Geometry check sheet. Reference: the model listing, model coordinates, mm. A direction names the side the tool comes from. Round coordinates to 2 decimals unless told otherwise and drop trailing zeros. Write each loop counter-clockwise with the first axis right and the second up, starting at its lowest first coordinate (ties: lowest second). Pieces come first, ordered by that corner, then holes. Notation, with made-up numbers: (81, -8.5) - (104, -8.5) arc R11 ccw to (104, 3.5) - close; hole circle Ø6 at (59, 6.5). An arc over 180 degrees is marked (long way). Return JSON: item names as keys, results as strings.
```python
from build123d import *

# Parameters (mm, degrees)
SKETCH1_R           = 23
SKETCH1_R_2         = 1.6
BOSS_EXTRUDE1_DEPTH = 10
SKETCH2_R           = 27.6
CUT_EXTRUDE1_DEPTH  = 7


with BuildPart() as part:
    # Sketch1 → Boss-Extrude1 (new body)
    with BuildSketch(Plane.XY):
        with BuildLine():
            ThreePointArc((-28.945945946, 19.675675676), (-35, 0), (-28.945945946, -19.675675676))
            ThreePointArc((-28.945945946, -19.675675676), (-28.600540614, -20.846499055), (-29, -22))
            ThreePointArc((-29, -22), (-28.535533906, -28.535533906), (-22, -29))
            ThreePointArc((-22, -29), (-20.846499055, -28.600540614), (-19.675675676, -28.945945946))
            ThreePointArc((-19.675675676, -28.945945946), (0, -35), (19.675675676, -28.945945946))
            ThreePointArc((19.675675676, -28.945945946), (20.846499055, -28.600540614), (22, -29))
            ThreePointArc((22, -29), (28.535533906, -28.535533906), (29, -22))
            ThreePointArc((29, -22), (28.600540614, -20.846499055), (28.945945946, -19.675675676))
            ThreePointArc((28.945945946, -19.675675676), (35, 0), (28.945945946, 19.675675676))
            ThreePointArc((28.945945946, 19.675675676), (28.600540614, 20.846499055), (29, 22))
            ThreePointArc((29, 22), (28.535533906, 28.535533906), (22, 29))
            ThreePointArc((22, 29), (20.846499055, 28.600540614), (19.675675676, 28.945945946))
            ThreePointArc((19.675675676, 28.945945946), (0, 35), (-19.675675676, 28.945945946))
            ThreePointArc((-19.675675676, 28.945945946), (-20.846499055, 28.600540614), (-22, 29))
            ThreePointArc((-22, 29), (-28.535533906, 28.535533906), (-29, 22))
            ThreePointArc((-29, 22), (-28.600540614, 20.846499055), (-28.945945946, 19.675675676))
        make_face()
        Circle(SKETCH1_R, mode=Mode.SUBTRACT)
        with Locations((-25, 25)):
            Circle(SKETCH1_R_2, mode=Mode.SUBTRACT)
        with Locations((25, 25)):
            Circle(SKETCH1_R_2, mode=Mode.SUBTRACT)
        with Locations((-25, -25)):
            Circle(SKETCH1_R_2, mode=Mode.SUBTRACT)
        with Locations((25, -25)):
            Circle(SKETCH1_R_2, mode=Mode.SUBTRACT)
    extrude(amount=BOSS_EXTRUDE1_DEPTH)

    # Sketch2 → Cut-Extrude1 (cut)
    with BuildSketch(Plane.XY.offset(10)):
        Circle(SKETCH2_R)
    extrude(amount=-CUT_EXTRUDE1_DEPTH, mode=Mode.SUBTRACT)


solid = part.part
```
(1) Release check for a two-part mould opening along Y. For faces 1 (the face through (0, 35, 5)), 2 (the face through (-28, 29, 5)), 3 (the face through (-29, -28, 5)), 4 (the face through (-20.86, -28.6, 4.93)) record: pulls with the +Y half, pulls with the -Y half, needs draft (parallel to the pull), parting line crosses it, or undercut.
Response values:
{"face 1": "pulls with the +Y half", "face 2": "undercut", "face 3": "undercut", "face 4": "pulls with the -Y half"}
(2) Section check C-C, the plane y = 25. Enter the section's corners in (x, z).
Response values:
{"outline": "(-30, 0) - (-26.6, 0) - (-26.6, 10) - (-30, 10) - close; (-23.4, 0) - (23.4, 0) - (23.4, 10) - (11.69, 10) - (11.69, 3) - (-11.69, 3) - (-11.69, 10) - (-23.4, 10) - close; (26.6, 0) - (30, 0) - (30, 10) - (26.6, 10) - close"}
(3) Gauge pin test, flat ends, axial feed: pin 1 (3 mm diameter, centred on x = 8.5, z = 3, fed in from -Y); pin 2 (2 mm diameter, centred on y = 13, z = 7.5, fed in from -X); pin 3 (1 mm diameter, centred on x = 1, y = -25.5, fed in from +Z). Record the tip position at first contact, or that the pin passes through.
Response values:
{"pin 1": "stops at y = -34.29", "pin 2": "stops at x = -32.88", "pin 3": "stops at z = 3"}
(4) Access from +Z, -Z, +X, -X, +Y, -Y to the whole of each face (thin tool, end or side, straight path). Record for faces 5 (the face through (-20.8, 28.6, 4.9)), 6 (the face through (-3.593, 27.365, 6.549)).
Response values:
{"face 5": "+Z, -Z, +Y", "face 6": "+Z"}
(5) Section check B-B, the plane y = 0. Enter the section's corners in (x, z), plus the area to 3 significant figures.
Response values:
{"outline": "(-35, 0) - (-23, 0) - (-23, 3) - (-27.6, 3) - (-27.6, 10) - (-35, 10) - close; (23, 0) - (35, 0) - (35, 10) - (27.6, 10) - (27.6, 3) - (23, 3) - close", "area": "176 mm^2"}
(6) Material ranges on line 1 along X through (y, z) = (0, 1.9); line 2 along X through (y, z) = (14.5, 8); line 3 along Y through (x, z) = (-25, 6), recorded low to high. Write a range as [from, to].
Response values:
{"line 1": "x = [-35, -23], [23, 35]", "line 2": "x = [-31.86, -23.48], [23.48, 31.86]", "line 3": "y = [-30, -26.6], [-23.4, -11.69], [11.69, 23.4], [26.6, 30]"}
(7) Section check A-A, the plane z = 2. Enter the section's corners in (x, y), plus the area to 3 significant figures.
Response values:
{"outline": "(-29, -22) arc R5 ccw to (-22, -29) arc R2 cw to (-19.68, -28.95) arc R35 ccw to (19.68, -28.95) arc R2 cw to (22, -29) arc R5 ccw to (29, -22) arc R2 cw to (28.95, -19.68) arc R35 ccw to (28.95, 19.68) arc R2 cw to (29, 22) arc R5 ccw to (22, 29) arc R2 cw to (19.68, 28.95) arc R35 ccw to (-19.68, 28.95) arc R2 cw to (-22, 29) arc R5 ccw to (-29, 22) arc R2 cw to (-28.95, 19.68) arc R35 ccw to (-28.95, -19.68) arc R2 cw to start; hole circle Ø3.2 at (-25, -25); hole circle Ø3.2 at (-25, 25); hole circle Ø46 at (0, 0); hole circle Ø3.2 at (25, -25); hole circle Ø3.2 at (25, 25)", "area": "2,330 mm^2"}
